The drawing under review shows one solid part. Ordinate dimensions are in mm from its lowest x, y, z. A direction names the side the tool comes from. Round coordinates to 2 decimals unless told otherwise and drop trailing zeros. Loops run counter-clockwise (first coordinate to the right, second up) from the corner with the lowest first, then second, coordinate; pieces in that order, holes last. Notation, with made-up numbers: M -40,-13.75 L 8,-13.75 A19 ccw 8,-6.75 Z; hole C 74,-18 d11. An arc over 180 degrees is marked long. Use a Markdown table: item, result.
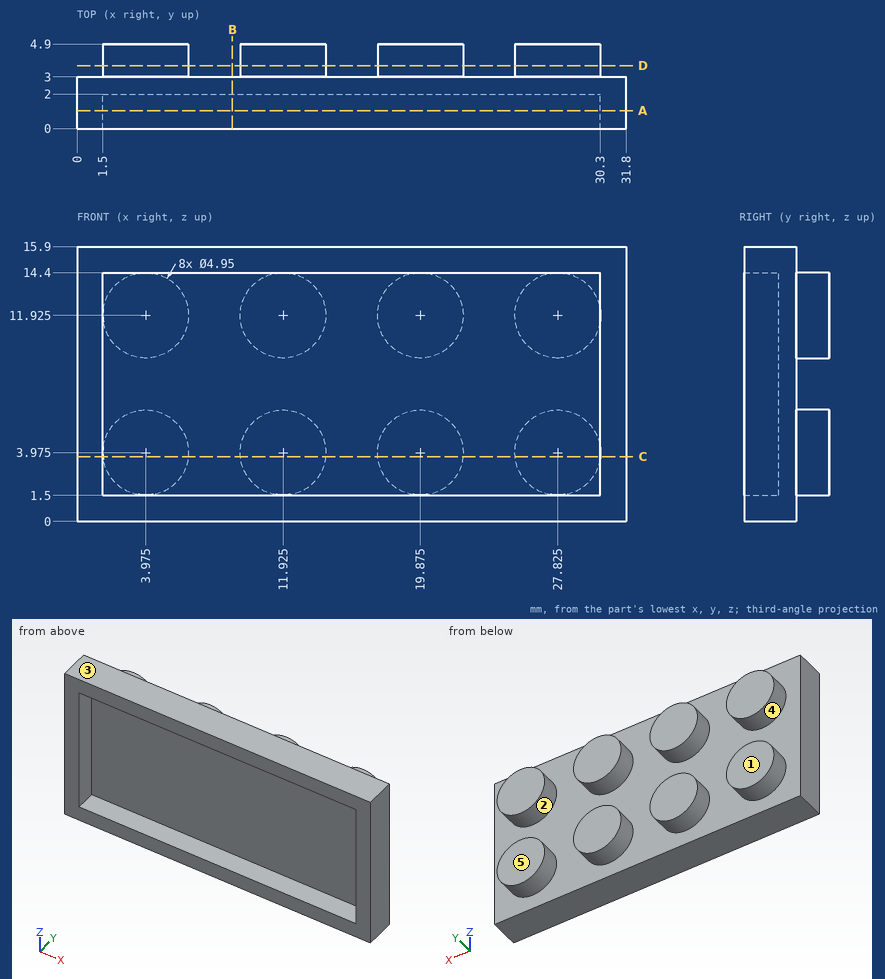
1. Take a section at D-D on y = 3.65. Give the boundary of the cut face in (x, z) (3 decimals), and give its area (3 significant figures).
Check values:
| item | result |
|---|---|
| outline | C 3.975,3.975 d4.95; C 3.975,11.925 d4.95; C 11.925,3.975 d4.95; C 11.925,11.925 d4.95; C 19.875,3.975 d4.95; C 19.875,11.925 d4.95; C 27.825,3.975 d4.95; C 27.825,11.925 d4.95 |
| area | 154 mm² |
2. Take a section at A-A on y = 1.05. Give the boundary of the cut face in (x, z), and give its area (3 significant figures).
Check values:
| item | result |
|---|---|
| outline | M 0,0 L 31.8,0 L 31.8,15.9 L 0,15.9 Z; hole M 1.5,1.5 L 30.3,1.5 L 30.3,14.4 L 1.5,14.4 Z |
| area | 134 mm² |
3. Take a section at C-C on z = 3.75. Give the boundary of the cut face in (x, y).
Check values:
| item | result |
|---|---|
| outline | M 0,0 L 1.5,0 L 1.5,2 L 30.3,2 L 30.3,0 L 31.8,0 L 31.8,3 L 30.29,3 L 30.29,4.9 L 25.36,4.9 L 25.36,3 L 22.34,3 L 22.34,4.9 L 17.41,4.9 L 17.41,3 L 14.39,3 L 14.39,4.9 L 9.46,4.9 L 9.46,3 L 6.44,3 L 6.44,4.9 L 1.51,4.9 L 1.51,3 L 0,3 Z |
4. Take a section at B-B on x = 9. Give the boundary of the cut face in (y, z), and give its area (3 significant figures).
Check values:
| item | result |
|---|---|
| outline | M 0,0 L 3,0 L 3,15.9 L 0,15.9 L 0,14.4 L 2,14.4 L 2,1.5 L 0,1.5 Z |
| area | 21.9 mm² |
5. Wall thickness on line 1 along X through (y, z) = (1.3, 10.75); line 2 along Z through (x, y) = (20, 3.8); line 3 along Z through (x, y) = (6.5, 0.8): over which ranges is each line inside the solid? List them lowest first. Write a range as from..to.
Check values:
| item | result |
|---|---|
| line 1 | x = 0..1.5, 30.3..31.8 |
| line 2 | z = 1.5..6.45, 9.45..14.4 |
| line 3 | z = 0..1.5, 14.4..15.9 |
6. The part is to be moulded in two halves that separate along Z. For the marked faces 1, 2 and 3, say which applies: pulls with the +Z half, pulls with the -Z half, needs draft (parallel to the pull), parting line crosses it, or undercut.
Check values:
| item | result |
|---|---|
| face 1 | needs draft |
| face 2 | undercut |
| face 3 | pulls with the +Z half |
7. Machinability: for the marked faces 4 and 5, which of the approach directions +Z, -Z, +X, -X, +Y, -Y give a long, thin tool a straight path to every point of the face, cutting with its end or side? Answer none if there is none.
Check values:
| item | result |
|---|---|
| face 4 | +Y |
| face 5 | +Z, -Z, +X, -X, +Y |
